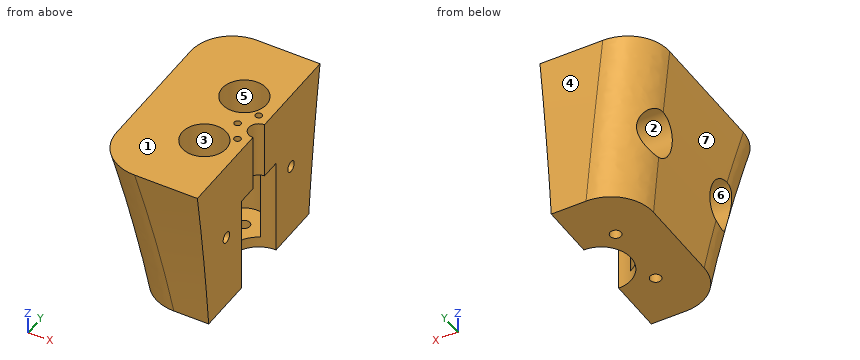
Autodesk Inventor part; units mm, degrees
ref_plane "Work Plane3" through (0, 0, 65) normal (0, 0, 1) x (1, 0, 0)
ref_plane "Work Plane4" through (0, 0, 35) normal (0, 0, 1) x (1, 0, 0)
ref_plane "Work Plane6" through (-12.5, 38.75, 70) normal (1, 0, 0) x (0, 1, 0)
sketch "Sketch1" plane through (0, 0, 0) normal (0, 0, 1) x (1, 0, 0)
  line L0 (0, 0) -> (70, 0)
  line L1 (70, 0) -> (70, 77.5)
  line L2 (70, 77.5) -> (0, 77.5)
  line L3 (0, 77.5) -> (0, 0)
  dimension "d0" = 70
  dimension "d1" = 77.5
extrude "Extrusion1" add sketch "Sketch1" along normal blind 70
sketch "Sketch3" plane through (0, 0, 70) normal (0, 0, 1) x (1, 0, 0)
  line L0 (0, 0) -> (70, 0)
  line L1 (70, 77.5) -> (0, 77.5)
  line L2 (70, 0) -> (35, 0)
  line L3 (35, 0) -> (35, 77.5)
  line L4 (35, 77.5) -> (70, 77.5)
  line L5 (70, 77.5) -> (70, 0)
extrude "Extrusion3" cut sketch "Sketch3" against normal through all
sketch "Sketch4" plane through (0, 77.5, 70) normal (0, 1, 0) x (1, 0, 0)
  line L0 (0, 70) -> (0, 0)
  line L1 (0, 0) -> (-12.5, 0)
  line L2 (35, 70) -> (0, 70)
  arc A0 (-12.5, 0) -> (0, 70) centre (-1137.8005, 237.0626) ccw
  line L3 (-12.5, -10) -> (35, -10) construction
  dimension "d9" = 1150
  dimension "d54" = 47.5
  dimension "d55" = 10
extrude "Extrusion4" add sketch "Sketch4" against normal blind 77.5
sketch "Sketch5" plane through (35, 0, 70) normal (1, 0, 0) x (0, 0, -1)
  line L0 (0, 77.5) -> (0, 86.25)
  line L1 (0, 0) -> (0, -8.75)
  line L2 (0, 0) -> (0, 77.5)
  line L3 (70, 77.5) -> (70, 0)
  arc A0 (0, 86.25) -> (70, 77.5) centre (177.5728, 1222.4577) ccw
  arc A1 (70, 0) -> (0, -8.75) centre (177.5728, -1144.9577) ccw
  line L4 (0, 77.5) -> (70, 77.5)
  line L5 (70, 0) -> (0, 0)
  line L6 (-10, 86.25) -> (-10, -8.75) construction
  point P0 (-10, 38.75)
  point P1 (0, 38.75)
  dimension "d14" = 1150
  dimension "d15" = 1150
  dimension "d52" = 10
  dimension "d53" = 95
extrude "Extrusion5" add sketch "Sketch5" against normal blind 55 contours L0 A0 L4 | L5 A1 L1
sketch "Sketch6" plane through (-20, 0, 0) normal (0, 1, 0) x (1, 0, 0)
  line L0 (20, 0) -> (0, 0)
  line L1 (0, -70) -> (0, 0)
  arc A0 (7.5, -70) -> (20, 0) centre (-1117.8005, 167.0626) ccw
  line L2 (7.5, -70) -> (0, -70)
extrude "Extrusion6" cut sketch "Sketch6" along normal through all both and the other way through all
fillet "Fillet3" radius 19.35 2 edges at (-5.7463, 81.368, 35.3063) (-5.7463, -3.868, 35.3063)
ref_plane "Work Plane3" through (0, 0, 65) normal (0, 0, 1) x (1, 0, 0)
sketch "Sketch24" plane through (0, 0, 65) normal (0, 0, 1) x (1, 0, 0)
  line L0 (35, 77.5) -> (35, 0)
  circle A0 centre (35, 38.75) radius 11.5
  point P0 (0, 0)
  dimension "d85" = 23
extrude "Extrusion20" cut sketch "Sketch24" against normal blind 9
sketch "Sketch26" plane through (0, 0, 70) normal (0, 0, 1) x (1, 0, 0)
  line L0 (35, 77.5) -> (35, 0)
  circle A0 centre (35, 38.75) radius 4.5
  point P0 (0, 0)
  dimension "d88" = 9
extrude "Extrusion21" cut sketch "Sketch26" against normal blind 50
ref_plane "Work Plane4" through (0, 0, 35) normal (0, 0, 1) x (1, 0, 0)
sketch "Sketch28" plane through (0, 0, 35) normal (0, 0, 1) x (1, 0, 0)
  line L0 (35, 43.25) -> (35, 34.25)
  circle A0 centre (35, 38.75) radius 11.5
  point P0 (0, 0)
  dimension "d92" = 23
extrude "Extrusion22" cut sketch "Sketch28" along normal blind 9
sketch "Sketch29" plane through (0, 0, 35) normal (0, 0, 1) x (1, 0, 0)
  line L0 (35, 43.25) -> (35, 34.25)
  circle A0 centre (35, 38.75) radius 11.5
  point P0 (0, 0)
  dimension "d96" = 23
extrude "Extrusion23" cut sketch "Sketch29" against normal through all
ref_plane "Work Plane6" through (-12.5, 38.75, 70) normal (1, 0, 0) x (0, 1, 0)
sketch "Sketch32" plane through (0, 0, 70) normal (0, 0, 1) x (1, 0, 0)
  circle A0 centre (19.5, 23.25) radius 2.5
  circle A1 centre (19.5, 54.25) radius 2.5
  line L0 (19.5, 54.25) -> (19.5, 23.25) construction
  arc A2 (35, 43.25) -> (35, 34.25) centre (35, 38.75) ccw
  line L1 (35, 86.25) -> (35, 43.25)
  point P0 (0, 0)
  point P1 (19.5, 38.75)
  dimension "d105" = 5
  dimension "d106" = 5
  dimension "d107" = 15.5
  dimension "d108" = 31
extrude "Extrusion26" cut sketch "Sketch32" against normal through all
sketch "Sketch33" plane through (0, 0, 70) normal (0, 0, 1) x (1, 0, 0)
  circle A0 centre (19.5, 54.25) radius 2.5
  circle A1 centre (19.5, 23.25) radius 2.5
  circle A2 centre (19.5, 54.25) radius 10
  circle A3 centre (19.5, 23.25) radius 10
  point P0 (0, 0)
  dimension "d111" = 20
  dimension "d112" = 20
extrude "Extrusion27" cut sketch "Sketch33" against normal blind 65
sketch "Sketch34" plane through (35, 50.25, 65) normal (1, 0, 0) x (0, 0, -1)
  circle A0 centre (31, 13.5) radius 2.5
  circle A1 centre (31, -36.5) radius 2.5
  line L0 (31, -36.5) -> (31, 13.5) construction
  line L1 (-5, -16) -> (-5, -7)
  line L2 (21, -7) -> (21, 0)
  point P0 (65, -50.25)
  point P1 (31, -11.5)
  point P2 (-5, -11.5)
  dimension "d115" = 5
  dimension "d116" = 5
  dimension "d117" = 50
  dimension "d118" = 10
extrude "Extrusion28" cut sketch "Sketch34" against normal through all
sketch "Sketch35" plane through (-12.5, 38.75, 70) normal (1, 0, 0) x (0, 1, 0)
  circle A0 centre (25, -36) radius 2.5
  circle A1 centre (-25, -36) radius 2.5
  circle A2 centre (25, -36) radius 10
  circle A3 centre (-25, -36) radius 10
  point P0 (-38.75, -70)
  dimension "d121" = 20
  dimension "d122" = 20
extrude "Extrusion29" cut sketch "Sketch35" along normal blind 40
sketch "Sketch36" plane through (0, 0, 44) normal (0, 0, -1) x (-1, 0, 0)
  arc A0 (-35, 34.25) -> (-35, 43.25) centre (-35, 38.75) ccw
  circle A1 centre (-35, 38.75) radius 13.5
  point P0 (0, 0)
  dimension "d125" = 27
extrude "Extrusion30" cut sketch "Sketch36" along normal through all
sketch "Sketch38" plane through (0, 0, 65) normal (0, 0, 1) x (1, 0, 0)
  arc A0 (35, 43.25) -> (35, 34.25) centre (35, 38.75) ccw
  line L0 (35, 27.25) -> (35, 34.25)
  arc A1 (35, 50.25) -> (35, 27.25) centre (35, 38.75) ccw
  line L1 (35, 43.25) -> (35, 50.25)
  point P0 (0, 0)
extrude "Extrusion32" add sketch "Sketch38" against normal blind 9
sketch "Sketch37" plane through (0, 0, 44) normal (0, 0, -1) x (-1, 0, 0)
  circle A0 centre (-25.475, 38.75) radius 1.5
  arc A1 (-35, 34.25) -> (-35, 43.25) centre (-35, 38.75) ccw
  circle A2 centre (-30.2375, 46.9989) radius 1.5
  circle A3 centre (-39.7625, 46.9989) radius 1.5
  circle A4 centre (-44.525, 38.75) radius 1.5
  circle A5 centre (-39.7625, 30.5011) radius 1.5
  circle A6 centre (-30.2375, 30.5011) radius 1.5
  point P0 (0, 0)
  dimension "d128" = 3
  dimension "d129" = 9.525
  dimension "d132" = 360
extrude "Extrusion31" cut sketch "Sketch37" against normal through all
properties part number "AA016" material "ABS Plastic"
Design review of the part built by this model. Coordinates are the model's own, in mm. Face numbers are marked on the shaded views. A direction names the side the tool comes from. Coordinates: 2 decimals unless noted, no trailing zeros. Loops run counter-clockwise (first coordinate to the right, second up) from the corner with the lowest first, then second, coordinate; pieces in that order, holes last. Notation, with made-up numbers: (35, 63.25) -> (53, 63.25) arc R23 ccw to (53, 101.25) -> close; hole circle Ø5 at (77, 40). An arc over 180 degrees is marked (long way). Answer as a JSON object with one key per item and string values.
Q1. Take a section at B-B on z = 34. Give the number of separate pieces and of enclosed holes in the cut face, plus the area to 3 significant figures.
Answer block:
{"separate pieces": "5", "enclosed holes": "0", "area": "1,340 mm^2"}
Q2. Clearance check with flat-ended pins moving along their axes: pin 1 Ø4 at (x, y) = (19, 29) entering from +Z; pin 2 Ø1 at (y, z) = (12, 31) entering from -X; pin 3 Ø1 at (x, z) = (11, 29.5) entering from -Y. State where each tip first meets the part, or that it passes through.
Answer block:
{"pin 1": "stops at z = 5", "pin 2": "stops at x = 27.5", "pin 3": "stops at y = -2.95"}
Q3. Take a section at A-A on y = 38.75. Give the boundary of the cut face in (x, z) (3 decimals), plus the area to 3 significant figures.
Answer block:
{"outline": "(-12.5, 70) arc R1149.999 cw to (0, 0) -> (21.5, 0) -> (21.5, 44) -> (23.975, 44) -> (23.975, 70) -> close; (26.975, 44) -> (30.5, 44) -> (30.5, 70) -> (26.975, 70) -> close", "area": "2,070 mm^2"}
Q4. The part is to be moulded in two halves that separate along Y. For the marked faces 1, 2, 3 and 4, say which applies: +Y half, -Y half, draft (parallel to the pull), parting line (faces both ways), or undercut.
Answer block:
{"face 1": "draft", "face 2": "undercut", "face 3": "undercut", "face 4": "+Y half"}
Q5. To check wall thickness, follow L1, parallel to Y at x = 31.75, z = 34; L2, parallel to Y at x = 14, z = 65; L3, parallel to Y at x = 19, z = 48. State the ranges of each line that lie inside material, in increasing order.
Answer block:
{"L1": "y = -3.71 to 11.25, 16.25 to 25.65, 51.85 to 61.25, 66.25 to 81.21", "L2": "y = -7.98 to 14.9, 31.6 to 45.9, 62.6 to 85.48", "L3": "y = -5.53 to 13.26, 33.24 to 44.26, 64.24 to 83.03"}
Q6. Tool access review of the marked faces 5, 6 and 7: name each direction out of +Z, -Z, +X, -X, +Y, -Y from which nothing blocks a thin tool from reaching the whole face with its end or side.
Answer block:
{"face 5": "+Z", "face 6": "-X", "face 7": "-Z, -X, +Y, -Y"}
